For this review, take the finished solid that the model builds, in its own axes (mm). Face numbers are marked on the shaded views. A direction names the side the tool comes from. Round coordinates to 2 decimals unless told otherwise and drop trailing zeros. Write each loop counter-clockwise with the first axis right and the second up, starting at its lowest first coordinate (ties: lowest second). Pieces come first, ordered by that corner, then holes. Notation, with made-up numbers: (-13.5, 5.5) - (14.5, 5.5) arc R15 cw to (14.5, 12.5) - close; hole circle Ø6 at (7.5, -28). An arc over 180 degrees is marked (long way). One line per item, written item: value. Start each with the question number.
Q1. Tool access review of the marked faces 1, 2, 3 and 4: name each direction out of +Z, -Z, +X, -X, +Y, -Y from which nothing blocks a thin tool from reaching the whole face with its end or side.
Q2. Mouldability with a two-part tool opening along Z and no side actions: class the marked faces 5, 6, 7 and 8 as +Z half, -Z half, draft (parallel to the pull), parting line (faces both ways), or undercut.
Q3. Add section C-C on y = 14.25. Write out the cut boundary in (x, z).
Q4. Add section D-D on y = 8. Write out the cut boundary in (x, z), and give its area (3 significant figures).
Q5. Add section A-A on x = 10. Write out the cut boundary in (y, z).
Q6. Add section B-B on z = 7.5. Write out the cut boundary in (x, y).
Q7. Clearance check with flat-ended pins moving along their axes: pin 1 Ø6 at (x, z) = (12, 4) entering from +Y; pin 2 Ø4.5 at (y, z) = (8, 7.5) entering from -X; pin 3 Ø2.5 at (y, z) = (11.5, 16) entering from +X. State where each tip first meets the part, or that it passes through.
Q8. For probe 1 along X at (y, z) = (13, 17); probe 2 along Y at (x, z) = (-2.3, 7.5); probe 3 along X at (y, z) = (-3.2, 7.5), list the stretches that pass through material, from the lowest coordinate up.
```python
from build123d import *

# Parameters (mm, degrees)
RESSALTO_EXTRUS_O2_DEPTH   = 15
ESBO_O4_R                  = 1.65
CORTE_EXTRUS_O1_DEPTH      = 1
CORTE_EXTRUS_O1_DEPTH_BACK = 25
ESBO_O5_R                  = 1.65
CORTE_EXTRUS_O2_DEPTH      = 15
ESBO_O6_R                  = 5.25
CORTE_EXTRUS_O3_DEPTH      = 1
ESBO_O7_R                  = 5.25
CORTE_EXTRUS_O4_DEPTH      = 1
RESSALTO_EXTRUS_O3_DEPTH   = 3
FILETE1_R                  = 5


with BuildPart() as part:
    # Esboço2 → Ressalto-extrusão2 (new body)
    with BuildSketch(Plane.XY):
        Polygon((0, 0), (20, 0), (20, -4), (-4, -4), (-4, 20), (0, 20), align=None)
    extrude(amount=RESSALTO_EXTRUS_O2_DEPTH)

    # Esboço4 → Corte-extrusão1 (cut, two sides)
    with BuildSketch(Plane.ZY.offset(4)) as corte_extrus_o1_sk:
        with Locations((7.5, 8)):
            Circle(ESBO_O4_R)
    extrude(amount=CORTE_EXTRUS_O1_DEPTH, mode=Mode.SUBTRACT)
    extrude(corte_extrus_o1_sk.sketch, amount=-CORTE_EXTRUS_O1_DEPTH_BACK, mode=Mode.SUBTRACT)

    # Esboço5 → Corte-extrusão2 (cut)
    with BuildSketch(Plane(origin=(0, 0, 0), x_dir=(1, 0, 0), z_dir=(0, 1, 0))):
        with Locations((10, -7.5)):
            Circle(ESBO_O5_R)
    extrude(amount=-CORTE_EXTRUS_O2_DEPTH, mode=Mode.SUBTRACT)

    # Esboço6 → Corte-extrusão3 (cut)
    with BuildSketch(Plane(origin=(0, 0, 0), x_dir=(1, 0, 0), z_dir=(0, 1, 0))):
        with Locations((10, -7.5)):
            Circle(ESBO_O6_R)
    extrude(amount=-CORTE_EXTRUS_O3_DEPTH, mode=Mode.SUBTRACT)

    # Esboço7 → Corte-extrusão4 (cut)
    with BuildSketch(Plane(origin=(0, 0, 0), x_dir=(0, 0, -1), z_dir=(1, 0, 0))):
        with Locations((-7.5, 8)):
            Circle(ESBO_O7_R)
    extrude(amount=-CORTE_EXTRUS_O4_DEPTH, mode=Mode.SUBTRACT)

    # Esboço9 → Ressalto-extrusão3 (add)
    with BuildSketch(Plane.XY.offset(15)):
        Polygon((20, -4), (-25.4, -4), (-25.4, 21), (0, 21), (0, 0), (20, 0), align=None)
        with BuildLine():
            Line((-22.1, 16), (-22.1, 1))
            ThreePointArc((-22.1, 1), (-20.4, -0.7), (-18.7, 1))
            Line((-18.7, 1), (-18.7, 16))
            ThreePointArc((-18.7, 16), (-20.4, 17.7), (-22.1, 16))
        make_face(mode=Mode.SUBTRACT)
        with BuildLine():
            Line((-9.3, 1), (-9.3, 16))
            ThreePointArc((-9.3, 16), (-11, 17.7), (-12.7, 16))
            Line((-12.7, 16), (-12.7, 1))
            ThreePointArc((-12.7, 1), (-11, -0.7), (-9.3, 1))
        make_face(mode=Mode.SUBTRACT)
    extrude(amount=RESSALTO_EXTRUS_O3_DEPTH)

    # Filete1
    filete1_edges = [part.edges().sort_by_distance(p)[0] for p in [
        (20, -2, 18),
        (-25.4, 21, 16.5),
        (-25.4, -4, 16.5),
        (20, -2, 0),
        (-2, 20, 0),
    ]]
    fillet(filete1_edges, radius=FILETE1_R)


solid = part.part
```
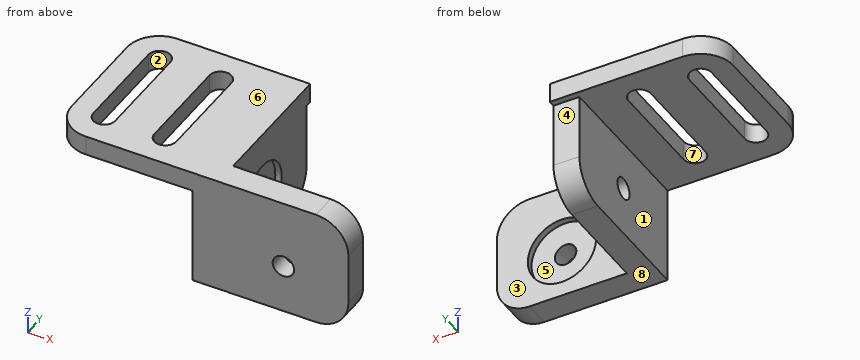
Result set:
1. face 1: -Z, -X, +Y, -Y
1. face 2: +Z, -Z
1. face 3: +Z, -Z, +X, +Y
1. face 4: -Z, +X, -X, +Y
2. face 5: undercut
2. face 6: +Z half
2. face 7: draft
2. face 8: -Z half
3. outline: (-25.4, 15) - (-22.1, 15) - (-22.1, 18) - (-25.4, 18) - close; (-18.7, 15) - (-12.7, 15) - (-12.7, 18) - (-18.7, 18) - close; (-9.3, 15) - (-4, 15) - (-4, 0) - (0, 0) - (0, 18) - (-9.3, 18) - close
4. outline: (-25.4, 15) - (-22.1, 15) - (-22.1, 18) - (-25.4, 18) - close; (-18.7, 15) - (-12.7, 15) - (-12.7, 18) - (-18.7, 18) - close; (-9.3, 15) - (-4, 15) - (-4, 9.15) - (-1, 9.15) - (-1, 12.75) - (0, 12.75) - (0, 18) - (-9.3, 18) - close; (-4, 0) - (0, 0) - (0, 2.25) - (-1, 2.25) - (-1, 5.85) - (-4, 5.85) - close
4. area: 95.4 mm^2
5. outline: (-4, 0) - (0, 0) - (0, 2.25) - (-1, 2.25) - (-1, 5.85) - (-4, 5.85) - close; (-4, 9.15) - (-1, 9.15) - (-1, 12.75) - (0, 12.75) - (0, 18) - (-4, 18) - close
6. outline: (-4, -4) - (8.35, -4) - (8.35, -1) - (4.75, -1) - (4.75, 0) - (0, 0) - (0, 2.75) - (-1, 2.75) - (-1, 6.35) - (-4, 6.35) - close; (-4, 9.65) - (-1, 9.65) - (-1, 13.25) - (0, 13.25) - (0, 20) - (-4, 20) - close; (11.65, -4) - (20, -4) - (20, 0) - (15.25, 0) - (15.25, -1) - (11.65, -1) - close
7. pin 1: stops at y = 0
7. pin 2: stops at x = -4
7. pin 3: stops at x = 0
8. probe 1: x = -25.4 to -22.1, -18.7 to -12.7, -9.3 to 0
8. probe 2: y = -4 to 6.35, 9.65 to 20
8. probe 3: x = -4 to 8.35, 11.65 to 20
